```python
from build123d import *

# Parameters (mm, degrees)
SKETCH2_W           = 1000
SKETCH2_H           = 663.636363636
BOSS_EXTRUDE1_DEPTH = 20
SKETCH3_W           = 948.152188742
SKETCH3_H           = 617.123435666
CUT_EXTRUDE1_DEPTH  = 10
CHAMFER1_SIZE       = 20


with BuildPart() as part:
    # Sketch2 → Boss-Extrude1 (new body)
    with BuildSketch(Plane.XY):
        Rectangle(SKETCH2_W, SKETCH2_H)
    extrude(amount=BOSS_EXTRUDE1_DEPTH)

    # Sketch3 → Cut-Extrude1 (cut)
    with BuildSketch(Plane.XY.offset(20)):
        Rectangle(SKETCH3_W, SKETCH3_H)
    extrude(amount=-CUT_EXTRUDE1_DEPTH, mode=Mode.SUBTRACT)

    # Chamfer1
    # the kernel refuses this chamfer: 20 mm, written as the material it adds along each edge
    with BuildSketch(Plane(origin=(-474.076094371, -308.561717833, 10), x_dir=(0, -0.0274958766105877, 0.9996219169112968), z_dir=(1, 0, 0))) as chamfer1_piece_1_section:
        Polygon((CHAMFER1_SIZE * 0.999621916911, -CHAMFER1_SIZE * 0.0274958766106), (-CHAMFER1_SIZE * 0.0274958766106, -CHAMFER1_SIZE * 0.999621916911), (0, 0), align=None)
    chamfer1_piece_1 = extrude(amount=948.152188741, mode=Mode.PRIVATE)
    chamfer1_piece_1 = split(chamfer1_piece_1, bisect_by=Plane(origin=(0, -300.783940055, 20), z_dir=(0, 0, -1)), keep=Keep.TOP, mode=Mode.PRIVATE)
    add(chamfer1_piece_1)
    with BuildSketch(Plane(origin=(-474.076094371, 308.561717833, 10), x_dir=(-0.0274958766105877, 0, 0.9996219169112968), z_dir=(0, -1, 0))) as chamfer1_piece_2_section:
        Polygon((CHAMFER1_SIZE * 0.999621916911, -CHAMFER1_SIZE * 0.0274958766106), (-CHAMFER1_SIZE * 0.0274958766106, -CHAMFER1_SIZE * 0.999621916911), (0, 0), align=None)
    chamfer1_piece_2 = extrude(amount=617.123435666, mode=Mode.PRIVATE)
    chamfer1_piece_2 = split(chamfer1_piece_2, bisect_by=Plane(origin=(-466.298316593, 0, 20), z_dir=(0, 0, -1)), keep=Keep.TOP, mode=Mode.PRIVATE)
    add(chamfer1_piece_2)
    with BuildSketch(Plane(origin=(474.076094371, 308.561717833, 10), x_dir=(0, 0.0274958766105877, 0.9996219169112968), z_dir=(-1, 0, 0))) as chamfer1_piece_3_section:
        Polygon((CHAMFER1_SIZE * 0.999621916911, -CHAMFER1_SIZE * 0.0274958766106), (-CHAMFER1_SIZE * 0.0274958766106, -CHAMFER1_SIZE * 0.999621916911), (0, 0), align=None)
    chamfer1_piece_3 = extrude(amount=948.152188741, mode=Mode.PRIVATE)
    chamfer1_piece_3 = split(chamfer1_piece_3, bisect_by=Plane(origin=(0, 300.783940055, 20), z_dir=(0, 0, -1)), keep=Keep.TOP, mode=Mode.PRIVATE)
    add(chamfer1_piece_3)
    with BuildSketch(Plane(origin=(474.076094371, -308.561717833, 10), x_dir=(0.0274958766105877, 0, 0.9996219169112968), z_dir=(0, 1, 0))) as chamfer1_piece_4_section:
        Polygon((CHAMFER1_SIZE * 0.999621916911, -CHAMFER1_SIZE * 0.0274958766106), (-CHAMFER1_SIZE * 0.0274958766106, -CHAMFER1_SIZE * 0.999621916911), (0, 0), align=None)
    chamfer1_piece_4 = extrude(amount=617.123435666, mode=Mode.PRIVATE)
    chamfer1_piece_4 = split(chamfer1_piece_4, bisect_by=Plane(origin=(466.298316593, 0, 20), z_dir=(0, 0, -1)), keep=Keep.TOP, mode=Mode.PRIVATE)
    add(chamfer1_piece_4)


solid = part.part
```
Geometry: final body of the model. Coordinates: model frame, mm. Round coordinates to 2 decimals unless told otherwise and drop trailing zeros. Order: outer loops, then holes, each group sorted by start corner. A loop starts at its lowest first (then second) coordinate and runs counter-clockwise, first axis right, second up. Notation, with made-up numbers: (65, 81) -> (77, 81) arc R16 ccw to (77, 91) -> close; hole circle Ø11 at (54, -39.5). An arc over 180 degrees is marked (long way). Use one line per item in the form item = value. Start each with the question number.
1. Line query: probe 1 along Z at (x, y) = (-306.5, -255.5); probe 2 along Y at (x, z) = (-166, 13.75); probe 3 along Y at (x, z) = (145, 11). Output: solid intervals per line, ascending.
2. Cut plane B-B (x = 377). Return the cut outline in (y, z).
3. Draft query along X for faces 1 (the face through (-6, 4, 10)), 2 (the face through (-7, -331.818, 10)), 3 (the face through (500, -5, 10)), 4 (the face through (-500, -5, 10)). Return one class per face: pulls with the +X half, pulls with the -X half, needs draft (parallel to the pull), parting line crosses it, or undercut.
4. Cut plane A-A (y = -66). Return the cut outline in (x, z).
5. Cut plane C-C (z = 15.75). Return the cut outline in (x, y), then the cut area to 3 significant figures.
Solution:
q1.probe_1 = 0 to 10
q1.probe_2 = -331.82 to -292.31, 292.31 to 331.82
q1.probe_3 = -331.82 to -289.56, 289.56 to 331.82
q2.outline = (-331.82, 0) -> (331.82, 0) -> (331.82, 20) -> (298.56, 20) -> (288.56, 10) -> (-288.56, 10) -> (-298.56, 20) -> (-331.82, 20) -> close
q3.face_1 = undercut
q3.face_2 = needs draft
q3.face_3 = pulls with the +X half
q3.face_4 = pulls with the -X half
q4.outline = (-500, 0) -> (500, 0) -> (500, 20) -> (464.08, 20) -> (454.08, 10) -> (-454.08, 10) -> (-464.08, 20) -> (-500, 20) -> close
q5.outline = (-500, -331.82) -> (500, -331.82) -> (500, 331.82) -> (-500, 331.82) -> close; hole (-459.83, -294.31) -> (459.83, -294.31) -> (459.83, 294.31) -> (-459.83, 294.31) -> close
q5.area = 122,000 mm^2
